Design review of the part built by this model. Coordinates are the model's own, in mm. A direction names the side the tool comes from. Give positions to 0.01 mm unless a question says otherwise; leave off trailing zeros. Order: outer loops, then holes, each group sorted by start corner. A loop starts at its lowest first (then second) coordinate and runs counter-clockwise, first axis right, second up. Notation, with made-up numbers: (69.5, 83) - (96.5, 83) arc R14 ccw to (96.5, 107) - close; hole circle Ø6 at (-2, -38). An arc over 180 degrees is marked (long way). Write each question's results on one line, items separated by ' | '. Start each with the question number.
```python
from build123d import *

# Parameters (mm, degrees)
SCHIZZO1_W                   = 77.07
SCHIZZO1_H                   = 15.19
ESTRUSIONE_ESTRUSIONE1_DEPTH = 5
TAGLIO_ESTRUSIONE1_DEPTH     = 6
SCHIZZO3_R                   = 1.5
TAGLIO_ESTRUSIONE2_DEPTH     = 6
SCHIZZO4_W                   = 5
SCHIZZO4_H                   = 15
ESTRUSIONE_ESTRUSIONE2_DEPTH = 3
TAGLIO_ESTRUSIONE3_DEPTH     = 6
SCHIZZO7_R                   = 0.25
TAGLIO_ESTRUSIONE4_DEPTH     = 10


with BuildPart() as part:
    # Schizzo1 → Estrusione-Estrusione1 (new body)
    with BuildSketch(Plane(origin=(0, 0, 0), x_dir=(0, 0, -1), z_dir=(1, 0, 0))):
        Rectangle(SCHIZZO1_W, SCHIZZO1_H)
    extrude(amount=ESTRUSIONE_ESTRUSIONE1_DEPTH)

    # Schizzo2 → Taglio-Estrusione1 (cut, through all)
    with BuildSketch(Plane(origin=(0, 0, 0), x_dir=(0, 0, -1), z_dir=(1, 0, 0))):
        Polygon((38.535, 7.595), (25.584422571, -7.595), (38.535, -7.595), align=None)
        Polygon((-38.535, 7.595), (-38.535, -7.595), (-20.718334969, -7.595), align=None)
    extrude(amount=TAGLIO_ESTRUSIONE1_DEPTH, mode=Mode.SUBTRACT)

    # Schizzo3 → Taglio-Estrusione2 (cut, through all)
    with BuildSketch(Plane(origin=(0, 0, 0), x_dir=(0, 0, -1), z_dir=(1, 0, 0))):
        with Locations((-18.535, 2.595)):
            Circle(SCHIZZO3_R)
        with Locations((18.535, 2.595)):
            Circle(SCHIZZO3_R)
    extrude(amount=TAGLIO_ESTRUSIONE2_DEPTH, mode=Mode.SUBTRACT)

    # Schizzo4 → Estrusione-Estrusione2 (add)
    with BuildSketch(Plane(origin=(0, 7.595, 0), x_dir=(1, 0, 0), z_dir=(0, 1, 0))):
        with Locations((2.5, 18.535)):
            Rectangle(SCHIZZO4_W, SCHIZZO4_H)
        with Locations((2.5, -18.535)):
            Rectangle(SCHIZZO4_W, SCHIZZO4_H)
    extrude(amount=ESTRUSIONE_ESTRUSIONE2_DEPTH)

    # Schizzo6 → Taglio-Estrusione3 (cut, through all)
    with BuildSketch(Plane(origin=(0, 0, 0), x_dir=(0, 0, -1), z_dir=(1, 0, 0))):
        Polygon((-1.25, -2.405), (-1.25, 1.395), (-2.75, 1.395), (-2.75, 3.795), (-1.25, 3.795), (-1.25, 7.595), (1.25, 7.595), (1.25, 3.795), (2.75, 3.795), (2.75, 1.395), (1.25, 1.395), (1.25, -2.405), align=None)
    extrude(amount=TAGLIO_ESTRUSIONE3_DEPTH, mode=Mode.SUBTRACT)

    # Schizzo7 → Taglio-Estrusione4 (cut)
    with BuildSketch(Plane(origin=(5, 0, 0), x_dir=(0, 0, -1), z_dir=(1, 0, 0))):
        with Locations((-2.75, 3.795)):
            Circle(SCHIZZO7_R)
        with Locations((2.75, 3.795)):
            Circle(SCHIZZO7_R)
    extrude(amount=-TAGLIO_ESTRUSIONE4_DEPTH, mode=Mode.SUBTRACT)


solid = part.part
```
Q1. Draft analysis for pull direction Y (two halves, no side actions). For faces 6 (the flat face through (2, 1.395, 2)), 7 (the flat face through (2, 7.595, 32)), 8 (the flat face through (2, 9, 26.035)), state which applies: pulls with the +Y half, pulls with the -Y half, needs draft (parallel to the pull), parting line crosses it, or undercut.
Q2. Add section D-D (z = 31). Give the boundary of the cut face in (x, y) (3 decimals).
Q3. For line 1 (Z direction, x = 4.7, y = 2); line 2 (Z direction, x = 0.5, y = 10.25) (3 decimals); line 3 (Y direction, x = 2.85, z = 8) (3 decimals), list the stretches that pass through material, from the lowest coordinate up. Write a range as [from, to].
Q4. Machinability: for faces 1 (the flat face through (2.465, 0.106, -32.15)), 2 (the flat face through (2, 9, -26.035)), 3 (the flat face through (2, 10.595, -19)), 4 (the flat face through (2, 7.595, -6)), 5 (the flat face through (2, 3.795, -2)), which of the approach directions +Z, -Z, +X, -X, +Y, -Y give a long, thin tool a straight path to every point of the face, cutting with its end or side? Answer none if there is none.
Q5. Add section C-C (z = -31.5). Give the boundary of the cut face in (x, y) (1 decimal), plus the area to 3 significant figures.
Q6. Add section B-B (y = 6). Give the boundary of the cut face in (x, z).
Q7. Insertion check: pin 1 Ø1.5 at (x, y) = (2, -5) entering from +Z; pin 2 Ø1.5 at (x, z) = (3.5, 4.5) entering from +Y (3 decimals); pin 3 Ø1 at (x, y) = (4, 1) entering from +Z. Each pin has a flat end and moves straight along its axis. Give the tip position at first contact, or say it passes through.
Q8. Add section A-A (x = 3.35). Give the boundary of the cut face in (y, z) (3 decimals).
Verdict:
1) face 6: undercut | face 7: pulls with the +Y half | face 8: needs draft
2) outline: (0, 1.171) - (5, 1.171) - (5, 7.595) - (0, 7.595) - close
3) line 1: z = [-33.76, -19.91], [-17.16, -2.75], [2.75, 17.16], [19.91, 31.97] | line 2: z = [-26.035, -11.035], [11.035, 26.035] | line 3: y = [-7.595, 7.595]
4) face 1: -Z, +X, -X, -Y | face 2: -Z, +X, -X, +Y | face 3: +Z, -Z, +X, -X, +Y | face 4: +X, -X, +Y | face 5: +X, -X
5) outline: (0, -0.7) - (5, -0.7) - (5, 7.6) - (0, 7.6) - close | area: 41.3 mm2
6) outline: (0, -37.18) - (5, -37.18) - (5, -1.25) - (0, -1.25) - close; (0, 1.25) - (5, 1.25) - (5, 36.66) - (0, 36.66) - close
7) pin 1: stops at z = 24.64 | pin 2: stops at y = 7.595 | pin 3: stops at z = 31.39
8) outline: (-7.595, -25.584) - (7.595, -38.535) - (7.595, -26.035) - (10.595, -26.035) - (10.595, -11.035) - (7.595, -11.035) - (7.595, -1.25) - (3.795, -1.25) - (3.795, -2.5) arc R0.25 cw (long way) to (3.545, -2.75) - (1.395, -2.75) - (1.395, -1.25) - (-2.405, -1.25) - (-2.405, 1.25) - (1.395, 1.25) - (1.395, 2.75) - (3.545, 2.75) arc R0.25 cw (long way) to (3.795, 2.5) - (3.795, 1.25) - (7.595, 1.25) - (7.595, 11.035) - (10.595, 11.035) - (10.595, 26.035) - (7.595, 26.035) - (7.595, 38.535) - (-7.595, 20.718) - close; hole circle Ø3 at (2.595, -18.535); hole circle Ø3 at (2.595, 18.535)
